Geometry: final body of the model. Coordinates: model frame, mm. Face numbers are marked on the shaded views. A direction names the side the tool comes from. Give positions to 0.01 mm unless a question says otherwise; leave off trailing zeros. Order: outer loops, then holes, each group sorted by start corner. A loop starts at its lowest first (then second) coordinate and runs counter-clockwise, first axis right, second up. Notation, with made-up numbers: (-8.5, 33.25) -> (49.5, 33.25) arc R16 ccw to (49.5, 54.25) -> close; hole circle Ø5 at (66.25, 31.25). An arc over 180 degrees is marked (long way). Answer in a Markdown table with one row per item. Add a question column.
Q1. Cut plane B-B on x = -21.5. Return the cut outline in (y, z).
Q2. Contact query for flat-ended pins moving along their axis: P1, Ø1.7, axis at x = -20, y = -15.5, coming from the -Z side; P2, Ø1.4, axis at x = -17, y = -15.5, coming from the +Z side; P3, Ø1.1, axis at y = -16, z = -40.5, coming from the +X side. Output: stop coordinate, or through.
Q3. Pull-direction query (X, two-part tool) for the marked faces 1, 2 and 3; classes: +X half, -X half, draft (parallel to the pull), parting line (faces both ways), or undercut.
Q4. Cut plane A-A on y = -15.25. Return the cut outline in (x, z), and give its area (3 significant figures).
Q5. Set-up query: the marked faces 4, 5, 6, 7 and 8. Return all of +Z, -Z, +X, -X, +Y, -Y with unobstructed straight access to the full face (end or side cutting, diameter ignored); none if empty.
Q6. Cut plane C-C on z = -38.75. Return the cut outline in (x, y), and give its area (3 significant figures).
Q7. Line query: line 1 along Z through (x, y) = (-21.5, -15.65); line 2 along X through (y, z) = (-15.7, -38.75); line 3 along Z through (x, y) = (2.25, -20.25). Output: solid intervals per line, ascending. Write a range as from..to.
Q8. Cut plane D-D on y = -18.5. Return the cut outline in (x, z), and give its area (3 significant figures).
from build123d import *

# Parameters (mm, degrees)
BOX013_W               = 3
BOX013_H               = 10
BOX013_DEPTH           = 2.85
BOX014_W               = 3
BOX014_H               = 10
BOX014_DEPTH           = 3.25
BOX012_W               = 4
BOX012_H               = 10
BOX012_DEPTH           = 1.4
CYLINDER012_R          = 0.7
CYLINDER012_DEPTH      = 10
CYLINDER012_ROLL_ANGLE = 90
CYLINDER013_R          = 0.7
CYLINDER013_DEPTH      = 10
CYLINDER013_ROLL_ANGLE = 90
BOX011_W               = 21
BOX011_H               = 4
BOX011_DEPTH           = 10
CHAMFER003_SIZE        = 3.8
CYLINDER014_R          = 1
CYLINDER014_DEPTH      = 5
CYLINDER014_ROLL_ANGLE = 90
BOX010_W               = 15.5
BOX010_H               = 2.7
BOX010_DEPTH           = 5
CHAMFER001_SIZE        = 1.5
CHAMFER002_SIZE        = 1.2
CHAMFER005_SIZE        = 2


with BuildPart() as cube008:
    # Box013 → Box013 (new body)
    with BuildSketch(Plane(origin=(-19, -19, -42), x_dir=(1, 0, 0), z_dir=(0, 0, 1))):
        with Locations((1.5, 5)):
            Rectangle(BOX013_W, BOX013_H)
    extrude(amount=BOX013_DEPTH)


with BuildPart() as fusion007008:
    # Box014 → Box014 (new body)
    with BuildSketch(Plane(origin=(-19, -19, -38.35), x_dir=(1, 0, 0), z_dir=(0, 0, 1))):
        with Locations((1.5, 5)):
            Rectangle(BOX014_W, BOX014_H)
    extrude(amount=BOX014_DEPTH)

    # Fusion007008: union Cube008
    add(cube008.part)


with BuildPart() as cube007:
    # Box012 → Box012 (new body)
    with BuildSketch(Plane(origin=(-7, -24.5, -39.3), x_dir=(1, 0, 0), z_dir=(0, 0, 1))):
        with Locations((2, 5)):
            Rectangle(BOX012_W, BOX012_H)
    extrude(amount=BOX012_DEPTH)


with BuildPart() as cylinder003:
    # Cylinder012 → Cylinder012 (new body)
    with BuildSketch(Plane.XY):
        Circle(CYLINDER012_R)
    extrude(amount=CYLINDER012_DEPTH)


with BuildPart() as cylinder003_1:
    # Cylinder012 roll: moved
    add(cylinder003.part.rotate(Axis((0, 0, 0), (1, 0, 0)), CYLINDER012_ROLL_ANGLE))


with BuildPart() as cylinder003_2:
    # Cylinder012 placement: moved
    add(cylinder003_1.part.moved(Location((-3, -14.5, -38.6))))


with BuildPart() as cylinder004:
    # Cylinder013 → Cylinder013 (new body)
    with BuildSketch(Plane.XY):
        Circle(CYLINDER013_R)
    extrude(amount=CYLINDER013_DEPTH)


with BuildPart() as cylinder004_1:
    # Cylinder013 roll: moved
    add(cylinder004.part.rotate(Axis((0, 0, 0), (1, 0, 0)), CYLINDER013_ROLL_ANGLE))


with BuildPart() as cylinder004_2:
    # Cylinder013 placement: moved
    add(cylinder004_1.part.moved(Location((-7, -14.5, -38.6))))


with BuildPart() as fusion007005:
    # Fusion007005 base: copy of Cylinder004
    add(cylinder004_2.part)

    # Fusion007005: union Cube007, Cylinder003
    add(cube007.part)
    add(cylinder003_2.part)


with BuildPart() as fusion007005_1:
    # Fusion007005 placement: moved
    add(fusion007005.part.moved(Location((7, 0, 0))))


with BuildPart() as fusion007006:
    # Fusion007006 base: copy of Cylinder004
    add(cylinder004_2.part)

    # Fusion007006: union Cube007, Cylinder003
    add(cube007.part)
    add(cylinder003_2.part)


with BuildPart() as chamfer003:
    # Box011 → Box011 (new body)
    with BuildSketch(Plane(origin=(-15, -21, -44), x_dir=(1, 0, 0), z_dir=(0, 0, 1))):
        with Locations((10.5, 2)):
            Rectangle(BOX011_W, BOX011_H)
    extrude(amount=BOX011_DEPTH)

    # Cut007: cut Fusion007006
    add(fusion007006.part, mode=Mode.SUBTRACT)

    # Cut008: cut Fusion007005
    add(fusion007005_1.part, mode=Mode.SUBTRACT)

    # Chamfer003
    chamfer003_edges = [chamfer003.edges().sort_by_distance(p)[0] for p in [
        (-15, -21, -39),
    ]]
    chamfer(chamfer003_edges, length=CHAMFER003_SIZE)


with BuildPart() as cylinder005:
    # Cylinder014 → Cylinder014 (new body)
    with BuildSketch(Plane.XY):
        Circle(CYLINDER014_R)
    extrude(amount=CYLINDER014_DEPTH)


with BuildPart() as cylinder005_1:
    # Cylinder014 roll: moved
    add(cylinder005.part.rotate(Axis((0, 0, 0), (1, 0, 0)), CYLINDER014_ROLL_ANGLE))


with BuildPart() as cylinder005_2:
    # Cylinder014 placement: moved
    add(cylinder005_1.part.moved(Location((-21.5, -13.5, -38.75))))


with BuildPart() as final_connectingrod:
    # Box010 → Box010 (new body)
    with BuildSketch(Plane(origin=(-24, -17.5, -41.25), x_dir=(1, 0, 0), z_dir=(0, 0, 1))):
        with Locations((7.75, 1.35)):
            Rectangle(BOX010_W, BOX010_H)
    extrude(amount=BOX010_DEPTH)

    # Cut009: cut Cylinder005
    add(cylinder005_2.part, mode=Mode.SUBTRACT)

    # Chamfer001
    chamfer001_edges = [final_connectingrod.edges().sort_by_distance(p)[0] for p in [
        (-24, -16.15, -36.25),
        (-24, -16.15, -41.25),
    ]]
    chamfer(chamfer001_edges, length=CHAMFER001_SIZE)

    # Chamfer002
    chamfer002_edges = [final_connectingrod.edges().sort_by_distance(p)[0] for p in [
        (-15.5, -17.5, -41.25),
        (-15.5, -17.5, -36.25),
    ]]
    chamfer(chamfer002_edges, length=CHAMFER002_SIZE)

    # Fusion007007: union Chamfer003
    add(chamfer003.part)

    # Chamfer005
    chamfer005_edges = [final_connectingrod.edges().sort_by_distance(p)[0] for p in [
        (-4.5, -17, -34),
        (-4.5, -17, -44),
    ]]
    chamfer(chamfer005_edges, length=CHAMFER005_SIZE)

    # Cut010: cut Fusion007008
    add(fusion007008.part, mode=Mode.SUBTRACT)


solid = final_connectingrod.part
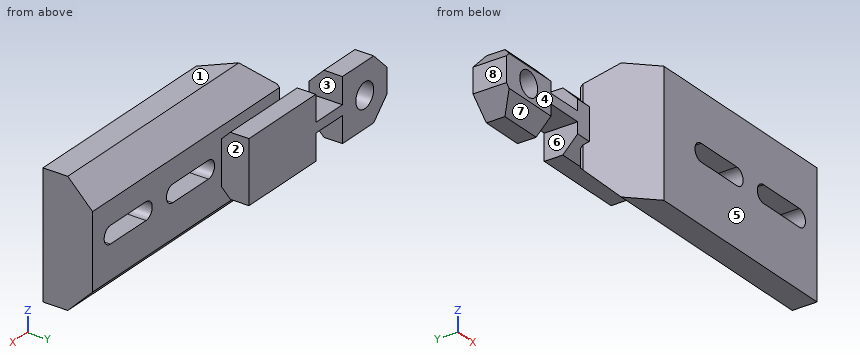
Completed:
| question | item | result |
|---|---|---|
| 1 | outline | (-17.5, -40.05) -> (-16.3, -41.25) -> (-14.8, -41.25) -> (-14.8, -39.75) -> (-17.5, -39.75) -> close; (-17.5, -37.75) -> (-14.8, -37.75) -> (-14.8, -36.25) -> (-16.3, -36.25) -> (-17.5, -37.45) -> close |
| 2 | P1 | stops at z = -41.25 |
| 2 | P2 | stops at z = -38.35 |
| 2 | P3 | stops at x = -8.5 |
| 3 | face 1 | draft |
| 3 | face 2 | +X half |
| 3 | face 3 | undercut |
| 4 | outline | (-24, -39.75) -> (-22.5, -41.25) -> (-19, -41.25) -> (-19, -39.15) -> (-16, -39.15) -> (-16, -41.25) -> (-8.5, -41.25) -> (-8.5, -36.25) -> (-16, -36.25) -> (-16, -38.35) -> (-19, -38.35) -> (-19, -36.25) -> (-22.5, -36.25) -> (-24, -37.75) -> close; hole circle Ø2 at (-21.5, -38.75) |
| 4 | area | 59.5 mm² |
| 5 | face 4 | +Z, -Z, -X, -Y |
| 5 | face 5 | +Z, -Z, +X, -X, -Y |
| 5 | face 6 | -Z, +Y, -Y |
| 5 | face 7 | -Z, -X, -Y |
| 5 | face 8 | +Z, -Z, -X, +Y, -Y |
| 6 | outline | (-24, -17.5) -> (-22.5, -17.5) -> (-22.5, -14.8) -> (-24, -14.8) -> close; (-20.5, -17.5) -> (-14.7, -17.5) -> (-11.2, -21) -> (-7.68, -21) -> (-7.68, -17) -> (-8.5, -17) -> (-8.5, -14.8) -> (-20.5, -14.8) -> close; (-2.32, -21) -> (-0.68, -21) -> (-0.68, -17) -> (-2.32, -17) -> close; (4.68, -21) -> (6, -21) -> (6, -17) -> (4.68, -17) -> close |
| 6 | area | 67.1 mm² |
| 7 | line 1 | z = -41.25..-39.75, -37.75..-36.25 |
| 7 | line 2 | x = -24..-22.5, -20.5..-8.5 |
| 7 | line 3 | z = -44..-39.3, -37.9..-34 |
| 8 | outline | (-13.7, -43.5) -> (6, -43.5) -> (6, -34.5) -> (-13.7, -34.5) -> close; hole (-7, -39.3) -> (-3, -39.3) arc R0.7 ccw to (-3, -37.9) -> (-7, -37.9) arc R0.7 ccw to start; hole (0, -39.3) -> (4, -39.3) arc R0.7 ccw to (4, -37.9) -> (0, -37.9) arc R0.7 ccw to start |
| 8 | area | 163 mm² |
